```python
from build123d import *

# Parameters (mm, degrees)
F2_W     = 13.43354
F2_H     = 47.182618
F3_DEPTH = 25


with BuildPart() as f1:
    # F0 (on Front) → F1 (revolve)
    with BuildSketch(Plane.XZ):
        Polygon((-42.259444, 64.114208), (-47.259444, 64.114208), (-35, 0), (-35, -25), (0, -25), (0, 0), (0, 5), (-30.956063, 5), align=None)
    revolve(axis=Axis((0, 0, -12.5), (0, 0, 1)))

    # F2 (on face) → F3 (cut)
    with BuildSketch(Plane.XY.offset(5)):
        with Locations((0, -1.463118)):
            Rectangle(F2_W, F2_H)
    extrude(amount=-F3_DEPTH, mode=Mode.SUBTRACT)


solid = f1.part
```
Model file for the job. Use its own axes, mm. A direction names the side the tool comes from. Give positions to 0.01 mm unless a question says otherwise; leave off trailing zeros. Write each loop counter-clockwise with the first axis right and the second up, starting at its lowest first coordinate (ties: lowest second). Pieces come first, ordered by that corner, then holes. Notation, with made-up numbers: (41, 63) -> (57, 63) arc R10 ccw to (57, 70) -> close; hole circle Ø8 at (-8.75, 43.5). An arc over 180 degrees is marked (long way). Use CSV: the item, a comma, the result in double quotes. Start each with the question number.
1) Cut at B-B on x = 0. List the corners of the cut face in (y, z).
2) Tool access for faces 1 (the cylindrical face through (28, 21, -13)), 2 (the flat face through (-35, 24, 64.114)), 3 (the flat face through (0, -1, -20)): list every direction of +Z, -Z, +X, -X, +Y, -Y with a clear straight run to the whole face (end or side of a thin tool).
3) Two-plate mould, pull along X, no slides. Class faces 4 (the flat face through (0, 0, -25)), 5 (the conical face through (-37.85, -11.92, 24.48)), 6 (the flat face through (0, -25.054, -7)): released by +X, released by -X, zero draft, split by the parting line, or undercut.
4) Pin check, flat tips, straight feed: P1, Ø12, axis at x = 31.5, z = 9, coming from the +Y side; P2, Ø12.5, axis at y = -7.5, z = -11, coming from the +X side; P3, Ø4, axis at x = -15, z = 46.5, coming from the +Y side; P4, Ø8, axis at x = 36, y = -35, coming from the +Z side. Stop position of each tip, or through.
5) Cut at D-D on z = 21. List the corners of the cut face in (x, y).
6) Cut at C-C on y = 0. List the corners of the cut face in (x, z), plus the area to 3 significant figures.
7) Cut at A-A on z = -15. List the corners of the cut face in (x, y), plus the area to 3 significant figures.
8) Drill centre lines: L1, parallel to X at y = 19.5, z = 40.5; L2, parallel to X at y = 13.5, z = 11; L3, parallel to Y at x = -5, z = 20. Where is each one in solid material? Low to high.
Final values:
1,outline,"(-47.26, 64.11) -> (-35, 0) -> (-35, -25) -> (35, -25) -> (35, 0) -> (47.26, 64.11) -> (42.26, 64.11) -> (30.96, 5) -> (22.13, 5) -> (22.13, -20) -> (-25.05, -20) -> (-25.05, 5) -> (-30.96, 5) -> (-42.26, 64.11) -> close"
2,face 1,"-Z"
2,face 2,"+Z, +X, -X, +Y, -Y"
2,face 3,"+Z"
3,face 4,"zero draft"
3,face 5,"split by the parting line"
3,face 6,"undercut"
4,P1,"stops at y = 26.64"
4,P2,"stops at x = 34.98"
4,P3,"stops at y = 42.04"
4,P4,"stops at z = 64.11"
5,outline,"circle Ø78.03 at (0, 0); hole circle Ø68.03 at (0, 0)"
6,outline,"(-47.26, 64.11) -> (-35, 0) -> (-35, -25) -> (35, -25) -> (35, 0) -> (47.26, 64.11) -> (42.26, 64.11) -> (30.96, 5) -> (6.72, 5) -> (6.72, -20) -> (-6.72, -20) -> (-6.72, 5) -> (-30.96, 5) -> (-42.26, 64.11) -> close"
6,area,"2,360 mm2"
7,outline,"circle Ø70 at (0, 0); hole (-6.72, -25.05) -> (6.72, -25.05) -> (6.72, 22.13) -> (-6.72, 22.13) -> close"
7,area,"3,210 mm2"
8,L1,"x = -38.04 to -32.32, 32.32 to 38.04"
8,L2,"x = -34.56 to -29.13, 29.13 to 34.56"
8,L3,"y = -38.5 to -33.45, 33.45 to 38.5"
